Build history of the part. All positions in model axes, mm. A direction names the side the tool comes from. Round coordinates to 2 decimals unless told otherwise and drop trailing zeros. Answer as a JSON object with one key per item and string values. Group by question number.
Item 1: Slice it at A-A, the plane z = 170. Give the number of separate pieces and of enclosed holes in the cut face, then the cut area to 3 significant figures.
Item 2: Flat gauge pins, fed straight in: pin 1 (0.8 mm diameter, centred on x = 1.5, z = 119.5, fed in from +Y); pin 2 (1.3 mm diameter, centred on y = 9, z = 52.5, fed in from -X); pin 3 (2 mm diameter, centred on y = -10.5, z = 135, fed in from +X); pin 4 (2 mm diameter, centred on x = -3, y = 16, fed in from -Z). Where does each tip first touch, or does it go through?
Item 3: Which spindle directions (+Z, -Z, +X, -X, +Y, -Y) get a long thin tool onto all of the face, cutting with end or side? Do faces 5 (the flat face through (10.107, 17, 99)), 6 (the flat face through (4.7, 4.7, 98.6)). Say none if no direction does.
Item 4: Two-plate mould, pull along Y, no slides. Class faces 1 (the flat face through (7, 20.356, 99)), 2 (the flat face through (-4.456, -4.02, 98.6)), 3 (the cylindrical face through (-0.167, 12.438, 98.6)), 4 (the flat face through (10.107, -17, 99)): +Y half, -Y half, draft (parallel to the pull), parting line (faces both ways), or undercut.
Item 5: Probe line 1 (Y direction, x = -7.25, z = 30.5); line 2 (X direction, y = -0.5, z = 186); line 3 (Y direction, x = -1, z = 88.5). List the from-to ranges inside material, lowest first. Write a range as from..to.
from build123d import *

# Parameters (mm, degrees)
SKETCH2_R           = 2.1
BOSS_EXTRUDE1_DEPTH = 200


with BuildPart() as part:
    # Sketch2 → Boss-Extrude1 (new body)
    with BuildSketch(Plane.XY):
        with BuildLine():
            Line((4.006804208, 10.145798499), (3.796804208, 10.355798499))
            Line((3.796804208, 10.355798499), (4.006804208, 10.565798499))
            Line((4.006804208, 10.565798499), (4.006804208, 13.195138327))
            Line((4.006804208, 13.195138327), (6.66746438, 15.855798499))
            Line((6.66746438, 15.855798499), (8.306804208, 15.855798499))
            Line((8.306804208, 15.855798499), (8.306804208, 13.480798499))
            Line((8.306804208, 13.480798499), (8.651804208, 13.480798499))
            Line((8.651804208, 13.480798499), (10.106804208, 14.935798499))
            Line((10.106804208, 14.935798499), (10.106804208, 19.855798499))
            ThreePointArc((10.106804208, 19.855798499), (9.960357598, 20.209351889), (9.606804208, 20.355798499))
            Line((9.606804208, 20.355798499), (4.686804208, 20.355798499))
            Line((4.686804208, 20.355798499), (3.231804208, 18.900798499))
            Line((3.231804208, 18.900798499), (3.231804208, 18.555798499))
            Line((3.231804208, 18.555798499), (5.606804208, 18.555798499))
            Line((5.606804208, 18.555798499), (5.606804208, 16.91645867))
            Line((5.606804208, 16.91645867), (2.946144036, 14.255798499))
            Line((2.946144036, 14.255798499), (0.316804208, 14.255798499))
            Line((0.316804208, 14.255798499), (0.106804208, 14.045798499))
            Line((0.106804208, 14.045798499), (-0.103195792, 14.255798499))
            Line((-0.103195792, 14.255798499), (-2.73253562, 14.255798499))
            Line((-2.73253562, 14.255798499), (-5.393195792, 16.91645867))
            Line((-5.393195792, 16.91645867), (-5.393195792, 18.555798499))
            Line((-5.393195792, 18.555798499), (-3.018195792, 18.555798499))
            Line((-3.018195792, 18.555798499), (-3.018195792, 18.900798499))
            Line((-3.018195792, 18.900798499), (-4.473195792, 20.355798499))
            Line((-4.473195792, 20.355798499), (-9.393195792, 20.355798499))
            ThreePointArc((-9.393195792, 20.355798499), (-9.746749183, 20.209351889), (-9.893195792, 19.855798499))
            Line((-9.893195792, 19.855798499), (-9.893195792, 14.935798499))
            Line((-9.893195792, 14.935798499), (-8.438195792, 13.480798499))
            Line((-8.438195792, 13.480798499), (-8.093195792, 13.480798499))
            Line((-8.093195792, 13.480798499), (-8.093195792, 15.855798499))
            Line((-8.093195792, 15.855798499), (-6.453855964, 15.855798499))
            Line((-6.453855964, 15.855798499), (-3.793195792, 13.195138327))
            Line((-3.793195792, 13.195138327), (-3.793195792, 10.565798499))
            Line((-3.793195792, 10.565798499), (-3.583195792, 10.355798499))
            Line((-3.583195792, 10.355798499), (-3.793195792, 10.145798499))
            Line((-3.793195792, 10.145798499), (-3.793195792, 7.51645867))
            Line((-3.793195792, 7.51645867), (-6.453855964, 4.855798499))
            Line((-6.453855964, 4.855798499), (-8.093195792, 4.855798499))
            Line((-8.093195792, 4.855798499), (-8.093195792, 7.230798499))
            Line((-8.093195792, 7.230798499), (-8.438195792, 7.230798499))
            Line((-8.438195792, 7.230798499), (-9.893195792, 5.775798499))
            Line((-9.893195792, 5.775798499), (-9.893195792, -5.064201501))
            Line((-9.893195792, -5.064201501), (-8.438195792, -6.519201501))
            Line((-8.438195792, -6.519201501), (-8.093195792, -6.519201501))
            Line((-8.093195792, -6.519201501), (-8.093195792, -4.144201501))
            Line((-8.093195792, -4.144201501), (-6.453855964, -4.144201501))
            Line((-6.453855964, -4.144201501), (-3.793195792, -6.804861673))
            Line((-3.793195792, -6.804861673), (-3.793195792, -9.434201501))
            Line((-3.793195792, -9.434201501), (-3.583195792, -9.644201501))
            Line((-3.583195792, -9.644201501), (-3.793195792, -9.854201501))
            Line((-3.793195792, -9.854201501), (-3.793195792, -12.48354133))
            Line((-3.793195792, -12.48354133), (-6.453855964, -15.144201501))
            Line((-6.453855964, -15.144201501), (-8.093195792, -15.144201501))
            Line((-8.093195792, -15.144201501), (-8.093195792, -12.769201501))
            Line((-8.093195792, -12.769201501), (-8.438195792, -12.769201501))
            Line((-8.438195792, -12.769201501), (-9.893195792, -14.224201501))
            Line((-9.893195792, -14.224201501), (-9.893195792, -19.144201501))
            ThreePointArc((-9.893195792, -19.144201501), (-9.746749183, -19.497754892), (-9.393195792, -19.644201501))
            Line((-9.393195792, -19.644201501), (-4.473195792, -19.644201501))
            Line((-4.473195792, -19.644201501), (-3.018195792, -18.189201501))
            Line((-3.018195792, -18.189201501), (-3.018195792, -17.844201501))
            Line((-3.018195792, -17.844201501), (-5.393195792, -17.844201501))
            Line((-5.393195792, -17.844201501), (-5.393195792, -16.204861673))
            Line((-5.393195792, -16.204861673), (-2.73253562, -13.544201501))
            Line((-2.73253562, -13.544201501), (-0.103195792, -13.544201501))
            Line((-0.103195792, -13.544201501), (0.106804208, -13.334201501))
            Line((0.106804208, -13.334201501), (0.316804208, -13.544201501))
            Line((0.316804208, -13.544201501), (2.946144036, -13.544201501))
            Line((2.946144036, -13.544201501), (5.606804208, -16.204861673))
            Line((5.606804208, -16.204861673), (5.606804208, -17.844201501))
            Line((5.606804208, -17.844201501), (3.231804208, -17.844201501))
            Line((3.231804208, -17.844201501), (3.231804208, -18.189201501))
            Line((3.231804208, -18.189201501), (4.686804208, -19.644201501))
            Line((4.686804208, -19.644201501), (9.606804208, -19.644201501))
            ThreePointArc((9.606804208, -19.644201501), (9.960357598, -19.497754892), (10.106804208, -19.144201501))
            Line((10.106804208, -19.144201501), (10.106804208, -14.224201501))
            Line((10.106804208, -14.224201501), (8.651804208, -12.769201501))
            Line((8.651804208, -12.769201501), (8.306804208, -12.769201501))
            Line((8.306804208, -12.769201501), (8.306804208, -15.144201501))
            Line((8.306804208, -15.144201501), (6.66746438, -15.144201501))
            Line((6.66746438, -15.144201501), (4.006804208, -12.48354133))
            Line((4.006804208, -12.48354133), (4.006804208, -9.854201501))
            Line((4.006804208, -9.854201501), (3.796804208, -9.644201501))
            Line((3.796804208, -9.644201501), (4.006804208, -9.434201501))
            Line((4.006804208, -9.434201501), (4.006804208, -6.804861673))
            Line((4.006804208, -6.804861673), (6.66746438, -4.144201501))
            Line((6.66746438, -4.144201501), (8.306804208, -4.144201501))
            Line((8.306804208, -4.144201501), (8.306804208, -6.519201501))
            Line((8.306804208, -6.519201501), (8.651804208, -6.519201501))
            Line((8.651804208, -6.519201501), (10.106804208, -5.064201501))
            Line((10.106804208, -5.064201501), (10.106804208, 5.775798499))
            Line((10.106804208, 5.775798499), (8.651804208, 7.230798499))
            Line((8.651804208, 7.230798499), (8.306804208, 7.230798499))
            Line((8.306804208, 7.230798499), (8.306804208, 4.855798499))
            Line((8.306804208, 4.855798499), (6.66746438, 4.855798499))
            Line((6.66746438, 4.855798499), (4.006804208, 7.51645867))
            Line((4.006804208, 7.51645867), (4.006804208, 10.145798499))
        make_face()
        with Locations((0.106804208, -9.644201501)):
            Circle(SKETCH2_R, mode=Mode.SUBTRACT)
        with Locations((0.106804208, 10.355798499)):
            Circle(SKETCH2_R, mode=Mode.SUBTRACT)
        Polygon((-6.13253562, -2.344201501), (-2.73253562, -5.744201501), (2.946144036, -5.744201501), (6.346144036, -2.344201501), (8.306804208, -2.344201501), (8.306804208, 3.055798499), (6.346144036, 3.055798499), (2.946144036, 6.455798499), (-2.73253562, 6.455798499), (-6.13253562, 3.055798499), (-8.093195792, 3.055798499), (-8.093195792, -2.344201501), align=None, mode=Mode.SUBTRACT)
    extrude(amount=BOSS_EXTRUDE1_DEPTH)


solid = part.part
Geometry says:
{
 "1": {"separate pieces": "1", "enclosed holes": "3", "area": "300 mm^2"},
 "2": {"pin 1": "stops at y = 14.26", "pin 2": "stops at x = -3.79", "pin 3": "stops at x = 4.01", "pin 4": "passes through"},
 "3": {"face 5": "+Z, -Z, +X, +Y, -Y", "face 6": "+Z, -Z"},
 "4": {"face 1": "+Y half", "face 2": "undercut", "face 3": "undercut", "face 4": "draft"},
 "5": {"line 1": "y = -19.64..-15.14, -4.14..-2.34, 3.06..4.86, 15.86..20.36", "line 2": "x = -9.89..-8.09, 8.31..10.11", "line 3": "y = -13.54..-11.43, -7.86..-5.74, 6.46..8.57, 12.14..14.26"}
}
